Geometry: final body of the model. Coordinates: model frame, mm. A direction names the side the tool comes from. Coordinates: 2 decimals unless noted, no trailing zeros. Order: outer loops, then holes, each group sorted by start corner. A loop starts at its lowest first (then second) coordinate and runs counter-clockwise, first axis right, second up. Notation, with made-up numbers: (31.25, -11) -> (63.25, -11) arc R15 cw to (63.25, -6) -> close; hole circle Ø4 at (89.25, -23). An arc over 180 degrees is marked (long way). Answer in a Markdown table with one row per item. Add a question column.
1) Section query B-B on z = 0. Return the cut outline in (x, y), then the cut area to 3 significant figures.
2) Pull-direction query (Z, two-part tool) for faces 1 (the face through (3, 0, -3)), 2 (the face through (-0.9, 0.8, 3.9)); classes: +Z half, -Z half, draft (parallel to the pull), parting line (faces both ways), or undercut.
3) Contact query for flat-ended pins moving along their axis: P1, Ø11.5, axis at x = -4, z = 4, coming from the +Y side; P2, Ø1.5, axis at y = 3, z = 6, coming from the +X side; P3, Ø3, axis at x = -10, y = 5.5, coming from the +Z side; P4, Ø6.5, axis at x = 0, z = 0, coming from the -Y side. Output: stop coordinate, or through.
4) Section query D-D on z = -5.25. Return the cut outline in (x, y), then the cut area to 3 significant figures.
5) Section query C-C on y = 7. Return the cut outline in (x, z).
6) Section query A-A on x = 0. Return the cut outline in (y, z).
7) Set-up query: faces 3 (the face through (5, 1.588, 0)), 4 (the face through (0, 8.588, 12)). Return all of +Z, -Z, +X, -X, +Y, -Y with unobstructed straight access to the full face (end or side cutting, diameter ignored); none if empty.
8) Ray query, line 1 (X direction, y = 4.25, z = 0); line 2 (X direction, y = 0.55, z = 0). Return the intervals inside material, ascending. Write a range as from..to.
```python
from build123d import *

# Parameters (mm, degrees)
SKETCH2_R           = 11.458333303
BOSS_EXTRUDE1_DEPTH = 1.5875
SKETCH5_R           = 13.045833303
BOSS_EXTRUDE4_DEPTH = 1.5875
SKETCH5_4_R         = 13.045833303
SKETCH5_4_R_2       = 11.458333303
BOSS_EXTRUDE5_DEPTH = 7
SKETCH6_R           = 4.0005
CUT_EXTRUDE1_DEPTH  = 2.5875


with BuildPart() as part:
    # Sketch2 → Boss-Extrude1 (new body)
    with BuildSketch(Plane(origin=(0, 0, 0), x_dir=(1, 0, 0), z_dir=(0, 1, 0))):
        Circle(SKETCH2_R)
    extrude(amount=BOSS_EXTRUDE1_DEPTH)

    # Sketch5 → Boss-Extrude4 (add)
    with BuildSketch(Plane(origin=(0, 1.5875, 0), x_dir=(1, 0, 0), z_dir=(0, 1, 0))):
        Circle(SKETCH5_R)
    extrude(amount=-BOSS_EXTRUDE4_DEPTH)

    # Sketch5_4 → Boss-Extrude5 (add)
    with BuildSketch(Plane(origin=(0, 1.5875, 0), x_dir=(1, 0, 0), z_dir=(0, 1, 0))):
        Circle(SKETCH5_4_R)
        Circle(SKETCH5_4_R_2, mode=Mode.SUBTRACT)
    extrude(amount=BOSS_EXTRUDE5_DEPTH)

    # Sketch6 → Cut-Extrude1 (cut, through all)
    with BuildSketch(Plane(origin=(0, 1.5875, 0), x_dir=(1, 0, 0), z_dir=(0, 1, 0))):
        Circle(SKETCH6_R)
    extrude(amount=-CUT_EXTRUDE1_DEPTH, mode=Mode.SUBTRACT)


solid = part.part
```
Result:
| question | item | result |
|---|---|---|
| 1 | outline | (-13.05, 0) -> (-4, 0) -> (-4, 1.59) -> (-11.46, 1.59) -> (-11.46, 8.59) -> (-13.05, 8.59) -> close; (4, 0) -> (13.05, 0) -> (13.05, 8.59) -> (11.46, 8.59) -> (11.46, 1.59) -> (4, 1.59) -> close |
| 1 | area | 50.9 mm2 |
| 2 | face 1 | draft |
| 2 | face 2 | undercut |
| 3 | P1 | y = 1.59 |
| 3 | P2 | x = 11.94 |
| 3 | P3 | z = 9.9 |
| 3 | P4 | through |
| 4 | outline | (-11.94, 0) -> (11.94, 0) -> (11.94, 8.59) -> (10.18, 8.59) -> (10.18, 1.59) -> (-10.18, 1.59) -> (-10.18, 8.59) -> (-11.94, 8.59) -> close |
| 4 | area | 62.5 mm2 |
| 5 | outline | circle Ø26.09 at (0, 0); hole circle Ø22.92 at (0, 0) |
| 6 | outline | (0, -13.05) -> (8.59, -13.05) -> (8.59, -11.46) -> (1.59, -11.46) -> (1.59, -4) -> (0, -4) -> close; (0, 4) -> (1.59, 4) -> (1.59, 11.46) -> (8.59, 11.46) -> (8.59, 13.05) -> (0, 13.05) -> close |
| 7 | face 3 | +Y |
| 7 | face 4 | +Z, -Z, +X, -X, +Y |
| 8 | line 1 | -13.05..-11.46, 11.46..13.05 |
| 8 | line 2 | -13.05..-4, 4..13.05 |
